CAD build for the part. Positions are in the model's coordinates, mm. Face numbers are marked on the shaded views. A direction names the side the tool comes from. Round coordinates to 2 decimals unless told otherwise and drop trailing zeros. Write each loop counter-clockwise with the first axis right and the second up, starting at its lowest first coordinate (ties: lowest second). Pieces come first, ordered by that corner, then holes. Notation, with made-up numbers: (59.25, -16) -> (104.25, -16) arc R20 ccw to (104.25, 0) -> close; hole circle Ø5 at (56, 0.25). An arc over 180 degrees is marked (long way). Answer in a Markdown table with one row per item. Add a question column.
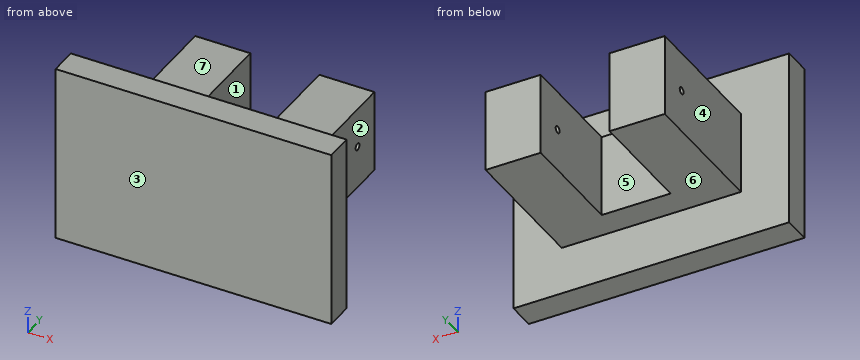
```python
from build123d import *

# Parameters (mm, degrees)
SKETCH_1_W          = 20
SKETCH_1_H          = 13
EXTRUDE_1_DEPTH     = 2
SKETCH_2_W          = 13
SKETCH_2_H          = 6
EXTRUDE_2_DEPTH     = 2
SKETCH_3_W          = 4
SKETCH_3_H          = 6
EXTRUDE_3_DEPTH     = 8
SKETCH_4_R          = 0.25
CUT_EXTRUDE_1_DEPTH = 23.21940351


with BuildPart() as part:
    # 草图1 → 凸台-拉伸1 (new body)
    with BuildSketch(Plane(origin=(0, 0, 0), x_dir=(1, 0, 0), z_dir=(0, 1, 0))):
        with Locations((-4.02027027, 2.300675676)):
            Rectangle(SKETCH_1_W, SKETCH_1_H)
    extrude(amount=EXTRUDE_1_DEPTH)

    # 草图2 → 凸台-拉伸2 (add)
    with BuildSketch(Plane(origin=(0, 2, 0), x_dir=(1, 0, 0), z_dir=(0, 1, 0))):
        with Locations((-4.02027027, 2.300675676)):
            Rectangle(SKETCH_2_W, SKETCH_2_H)
    extrude(amount=EXTRUDE_2_DEPTH)

    # 草图3 → 凸台-拉伸3 (add)
    with BuildSketch(Plane(origin=(0, 4, 0), x_dir=(1, 0, 0), z_dir=(0, 1, 0))):
        with Locations((-8.52027027, 2.300675676)):
            Rectangle(SKETCH_3_W, SKETCH_3_H)
        with Locations((0.47972973, 2.300675676)):
            Rectangle(SKETCH_3_W, SKETCH_3_H)
    extrude(amount=EXTRUDE_3_DEPTH)

    # 草图4 → 切除-拉伸1 (cut, through all)
    with BuildSketch(Plane.ZY.offset(10.52027027)):
        with Locations((-2.187687032, 9.784017998)):
            Circle(SKETCH_4_R)
    extrude(amount=-CUT_EXTRUDE_1_DEPTH, mode=Mode.SUBTRACT)


solid = part.part
```
Item 1: Saw through at A-A on y = 6.25. Give the cut face in (x, z).
Item 2: Tool access for the marked faces 5, 6 and 7: list every direction of +Z, -Z, +X, -X, +Y, -Y with a clear straight run to the whole face (end or side of a thin tool).
Item 3: Saw through at B-B on x = -6. Give the cut face in (y, z).
Item 4: Two-plate mould, pull along X, no slides. Class the marked faces 1, 2, 3 and 4: +X half, -X half, draft (parallel to the pull), parting line (faces both ways), or undercut.
Item 5: Saw through at C-C on z = 2.25. Give the cut face in (x, y).
Item 6: Saw through at D-D on x = 0.5. Give the cut face in (y, z).
Item 7: Drill centre lines: probe 1 along X at (y, z) = (6.25, 0); probe 2 along Z at (x, y) = (-0.75, 10.25); probe 3 along Y at (x, z) = (-11.75, 1.5). Where is each one in solid material? Low to high.
Item 8: Pin check, flat tips, straight feed: pin 1 (6.5 mm diameter, centred on y = 7.5, z = -3.5, fed in from +X); pin 2 (1.8 mm diameter, centred on y = 9.5, z = -2, fed in from -X); pin 3 (3 mm diameter, centred on x = -2.5, y = 9.5, fed in from +Z). Stop position of each tip, or through.
Recorded:
| question | item | result |
|---|---|---|
| 1 | outline | (-10.52, -5.3) -> (-6.52, -5.3) -> (-6.52, 0.7) -> (-10.52, 0.7) -> close; (-1.52, -5.3) -> (2.48, -5.3) -> (2.48, 0.7) -> (-1.52, 0.7) -> close |
| 2 | face 5 | +Z, -Z, +Y |
| 2 | face 6 | -Z, +X, -X, +Y |
| 2 | face 7 | +Z, +X, -X, +Y |
| 3 | outline | (0, -8.8) -> (2, -8.8) -> (2, -5.3) -> (4, -5.3) -> (4, 0.7) -> (2, 0.7) -> (2, 4.2) -> (0, 4.2) -> close |
| 4 | face 1 | undercut |
| 4 | face 2 | +X half |
| 4 | face 3 | draft |
| 4 | face 4 | -X half |
| 5 | outline | (-14.02, 0) -> (5.98, 0) -> (5.98, 2) -> (-14.02, 2) -> close |
| 6 | outline | (0, -8.8) -> (2, -8.8) -> (2, -5.3) -> (12, -5.3) -> (12, 0.7) -> (2, 0.7) -> (2, 4.2) -> (0, 4.2) -> close; hole circle Ø0.5 at (9.78, -2.19) |
| 7 | probe 1 | -10.52 to -6.52, -1.52 to 2.48 |
| 7 | probe 2 | -5.3 to 0.7 |
| 7 | probe 3 | 0 to 2 |
| 8 | pin 1 | x = 2.48 |
| 8 | pin 2 | x = -10.52 |
| 8 | pin 3 | z = 0.7 |
